For this review, use the dimensioned drawing (mm, ordinates from the lowest corner) and the shaded views. Round coordinates to 2 decimals unless told otherwise and drop trailing zeros. Loops run counter-clockwise (first coordinate to the right, second up) from the corner with the lowest first, then second, coordinate; pieces in that order, holes last. Notation, with made-up numbers: M 83,-24.5 L 90,-24.5 A18 cw 90,9.5 Z; hole C 39,6 d11. An arc over 180 degrees is marked long. Use a Markdown table: item, result. Add a question column.
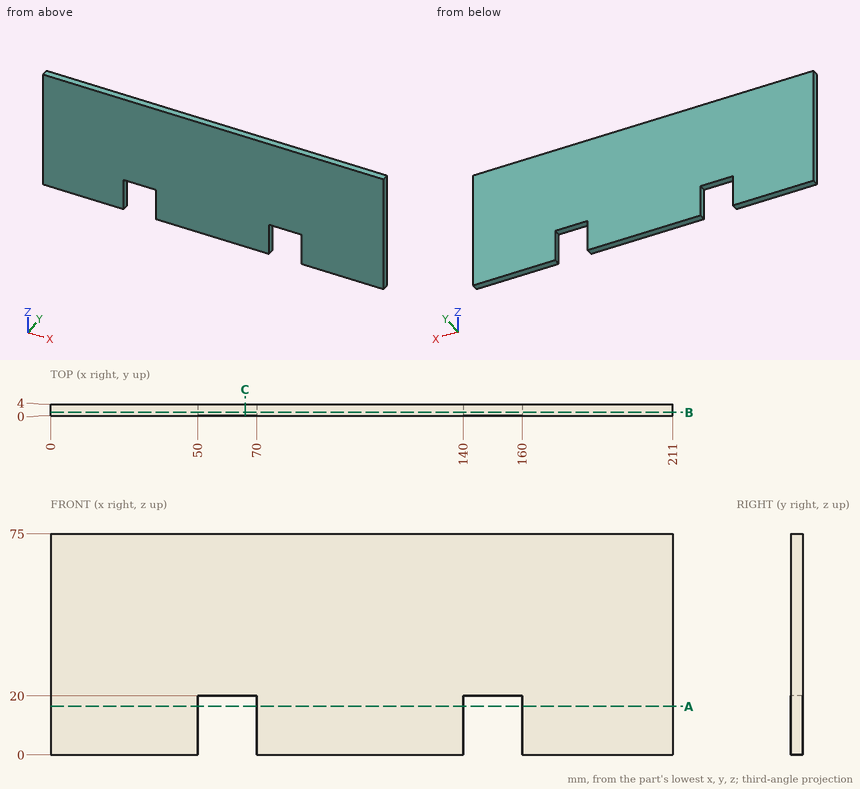
(1) Consider section C-C, the plane x = 66. Give the boundary of the cut face in (y, z).
(2) To check wall thickness, follow probe 1 along X at (y, z) = (0.8, 5); probe 2 along Z at (x, y) = (58, 1.7). State the ranges of each line that lie inside material, in increasing order.
(3) Insertion check: pin 1 Ø2 at (x, y) = (63.5, 2) entering from -Z. The pin has a flat end and moves straight along its axis. Give the tip position at first contact, or say it passes through.
(4) Consider section B-B, the plane y = 1.15. Give the boundary of the cut face in (x, z).
(5) Consider section A-A, the plane z = 16.5. Give the boundary of the cut face in (x, y), then the cut area to 3 significant figures.
Found:
| question | item | result |
|---|---|---|
| 1 | outline | M 0,20 L 4,20 L 4,75 L 0,75 Z |
| 2 | probe 1 | x = 0 to 50, 70 to 140, 160 to 211 |
| 2 | probe 2 | z = 20 to 75 |
| 3 | pin 1 | stops at z = 20 |
| 4 | outline | M 0,0 L 50,0 L 50,20 L 70,20 L 70,0 L 140,0 L 140,20 L 160,20 L 160,0 L 211,0 L 211,75 L 0,75 Z |
| 5 | outline | M 0,0 L 50,0 L 50,4 L 0,4 Z; M 70,0 L 140,0 L 140,4 L 70,4 Z; M 160,0 L 211,0 L 211,4 L 160,4 Z |
| 5 | area | 684 mm^2 |
